```python
from build123d import *

# Parameters (mm, degrees)
SKETCH_1_W          = 3
SKETCH_1_H          = 27
SKETCH_1_H_2        = 3
SKETCH_1_W_2        = 17
EXTRUDE_1_DEPTH     = 30
SKETCH_2_R          = 2
CUT_EXTRUDE_1_DEPTH = 10
CUT_EXTRUDE_2_DEPTH = 10
FILLET_1_R          = 3


with BuildPart() as part:
    # 草图1 → 凸台-拉伸1 (new body)
    with BuildSketch(Plane(origin=(0, 0, 0), x_dir=(1, 0, 0), z_dir=(0, 1, 0))):
        with Locations((0, 1.5)):
            Rectangle(SKETCH_1_W, SKETCH_1_H)
        with Locations((0, -13.5)):
            Rectangle(SKETCH_1_W, SKETCH_1_H_2)
        with Locations((10, -13.5)):
            Rectangle(SKETCH_1_W_2, SKETCH_1_H_2)
    extrude(amount=EXTRUDE_1_DEPTH)

    # 草图2 → 切除-拉伸1 (cut)
    with BuildSketch(Plane.XY.offset(15)):
        with Locations((11.5, 21.35)):
            Circle(SKETCH_2_R)
        with Locations((11.5, 8.65)):
            Circle(SKETCH_2_R)
        with Locations((11.5, -4.05)):
            Circle(SKETCH_2_R)
    extrude(amount=-CUT_EXTRUDE_1_DEPTH, mode=Mode.SUBTRACT)

    # 草图3 → 切除-拉伸2 (cut)
    with BuildSketch(Plane.ZY.offset(1.5)):
        with BuildLine():
            Line((-3, 24), (-3, 6))
            ThreePointArc((-3, 6), (-7, 2), (-11, 6))
            Line((-11, 6), (-11, 24))
            ThreePointArc((-11, 24), (-7, 28), (-3, 24))
        make_face()
    extrude(amount=-CUT_EXTRUDE_2_DEPTH, mode=Mode.SUBTRACT)

    # 圆角1
    fillet_1_edges = [part.edges().sort_by_distance(p)[0] for p in [
        (18.5, 0, 13.5),
        (18.5, 30, 13.5),
        (0, 30, -15),
        (0, 0, -15),
    ]]
    fillet(fillet_1_edges, radius=FILLET_1_R)


solid = part.part
```
Part model, mm, in its own coordinate system. A direction names the side the tool comes from. Round coordinates to 2 decimals unless told otherwise and drop trailing zeros. Write each loop counter-clockwise with the first axis right and the second up, starting at its lowest first coordinate (ties: lowest second). Pieces come first, ordered by that corner, then holes.
Item 1: Two-plate mould, pull along X, no slides. Class faces 4 (the cylindrical face through (0, 2, -7)), 5 (the cylindrical face through (17.6, 29.14, 13.48)), 6 (the cylindrical face through (9.913, 20.133, 13.521)), 7 (the flat face through (-1.5, 15, 3)): +X half, -X half, draft (parallel to the pull), parting line (faces both ways), or undercut.
Results:
face 4: draft
face 5: +X half
face 6: undercut
face 7: -X half
Item 2: Cut at A-A, the plane y = 11.5. Give the cut face in (x, z), plus the area to 3 significant figures.
Results:
outline: (-1.5, -15) - (1.5, -15) - (1.5, -11) - (-1.5, -11) - close; (-1.5, -3) - (1.5, -3) - (1.5, 12) - (18.5, 12) - (18.5, 15) - (-1.5, 15) - close
area: 117 mm2
Item 3: Probe L1, parallel to Y at x = 11.5, z = 13.35; L2, parallel to Z at x = 7.75, y = 6.5; L3, parallel to X at y = 27.5, z = -12.5. List the from-to ranges inside material, lowest first.
Results:
L1: y = 0 to 6.65, 10.65 to 19.35, 23.35 to 30
L2: z = 12 to 15
L3: x = -1.5 to 1.5
Item 4: Cut at B-B, the plane x = 11.5. Give the cut face in (y, z), plus the area to 3 significant figures.
Results:
outline: (0, 12) - (6.65, 12) - (6.65, 15) - (0, 15) - close; (10.65, 12) - (19.35, 12) - (19.35, 15) - (10.65, 15) - close; (23.35, 12) - (30, 12) - (30, 15) - (23.35, 15) - close
area: 66.0 mm2
Item 5: Cut at C-C, the plane z = -7. Give the cut face in (x, y).
Results:
outline: (-1.5, 0) - (1.5, 0) - (1.5, 2) - (-1.5, 2) - close; (-1.5, 28) - (1.5, 28) - (1.5, 30) - (-1.5, 30) - close
Item 6: Which spindle directions (+Z, -Z, +X, -X, +Y, -Y) get a long thin tool onto all of the face, cutting with end or side? Do faces 1 (the flat face through (0, 15, -15)), 2 (the flat face through (0, 15, -11)), 3 (the flat face through (1.5, 15, 2)). Say none if no direction does.
Results:
face 1: -Z, +X, -X, +Y, -Y
face 2: +X, -X
face 3: -Z, +X, +Y, -Y
Item 7: Cut at D-D, the plane y = 7.5. Give the cut face in (x, z), plus the area to 3 significant figures.
Results:
outline: (-1.5, -15) - (1.5, -15) - (1.5, -11) - (-1.5, -11) - close; (-1.5, -3) - (1.5, -3) - (1.5, 12) - (9.86, 12) - (9.86, 15) - (-1.5, 15) - close; (13.14, 12) - (18.5, 12) - (18.5, 15) - (13.14, 15) - close
area: 107 mm2
Item 8: Drop flat-ended pins along their axis: pin 1 Ø5 at (y, z) = (13, -2) entering from +X; pin 2 Ø5 at (x, y) = (8.5, 17.5) entering from -Z. Give the stop position or say it passes through.
Results:
pin 1: stops at x = 1.5
pin 2: stops at z = 12
